from build123d import *

# Parameters (mm, degrees)
F1_DEPTH = 19.05
F2_R     = 50.8
F3_R     = 25.4
F4_R     = 12.7


with BuildPart() as f1:
    # F0 (on Top) → F1 (new body)
    with BuildSketch(Plane.XY):
        Polygon((203.2, 0), (0, 0), (-101.6, 0), (-101.6, -355.6), (-50.8, -355.6), (0, -50.8), (203.2, -50.8), (254, -355.6), (304.8, -355.6), (304.8, 0), align=None)
    extrude(amount=F1_DEPTH)

    # F2
    f2_edges = [f1.edges().sort_by_distance(p)[0] for p in [
        (-101.6, 0, 9.525),
        (304.8, 0, 9.525),
    ]]
    fillet(f2_edges, radius=F2_R)

    # F3
    f3_edges = [f1.edges().sort_by_distance(p)[0] for p in [
        (-101.6, -355.6, 9.525),
        (-50.8, -355.6, 9.525),
        (304.8, -355.6, 9.525),
        (254, -355.6, 9.525),
    ]]
    fillet(f3_edges, radius=F3_R)

    # F4
    f4_edges = [f1.edges().sort_by_distance(p)[0] for p in [
        (203.2, -50.8, 9.525),
        (0, -50.8, 9.525),
    ]]
    fillet(f4_edges, radius=F4_R)


solid = f1.part
Verification items for the finished model (mm, model axes). A direction names the side the tool comes from. Coordinates: 2 decimals unless noted, no trailing zeros. Order: outer loops, then holes, each group sorted by start corner. A loop starts at its lowest first (then second) coordinate and runs counter-clockwise, first axis right, second up. Notation, with made-up numbers: M 13,78 L 69,78 A19 ccw 69,90 Z; hole C 39.25,71.5 d2. An arc over 180 degrees is marked long. Write each question's results on one line, items separated by ' | '.
1) Scan lines: line 1 along X through (y, z) = (-206.5, 3.5); line 2 along X through (y, z) = (-109, 9); line 3 along Y through (x, z) = (123, 14.75). Record each from-to range of solid material in increasing order. Write a range as [from, to].
Solved:
line 1: x = [-101.6, -25.95], [229.15, 304.8] | line 2: x = [-101.6, -9.7], [212.9, 304.8] | line 3: y = [-50.8, 0]
2) Section check C-C on x = -37.5. Record the cut outline in (y, z).
Solved:
outline: M -275.8,0 L 0,0 L 0,19.05 L -275.8,19.05 Z
3) Gauge pin test, flat end, axial feed: pin 1 Ø5.5 at (x, z) = (62, 12) entering from -Y. Record the tip position at first contact, or that the pin passes through.
Solved:
pin 1: stops at y = -50.8
4) Section check D-D on y = -173. Record the cut outline in (x, z).
Solved:
outline: M -101.6,0 L -20.37,0 L -20.37,19.05 L -101.6,19.05 Z; M 223.57,0 L 304.8,0 L 304.8,19.05 L 223.57,19.05 Z
5) Section check B-B on z = 13.25. Record the cut outline in (x, y).
Solved:
outline: M -101.6,-330.2 A25.4 ccw -76.2,-355.6 L -72.32,-355.6 A25.4 ccw -47.26,-334.38 L -1.77,-61.41 A12.7 cw 10.76,-50.8 L 192.44,-50.8 A12.7 cw 204.97,-61.41 L 250.46,-334.38 A25.4 ccw 275.52,-355.6 L 279.4,-355.6 A25.4 ccw 304.8,-330.2 L 304.8,-50.8 A50.8 ccw 254,0 L -50.8,0 A50.8 ccw -101.6,-50.8 Z
6) Section check A-A on y = -269.5. Record the cut outline in (x, z).
Solved:
outline: M -101.6,0 L -36.45,0 L -36.45,19.05 L -101.6,19.05 Z; M 239.65,0 L 304.8,0 L 304.8,19.05 L 239.65,19.05 Z
7) Release check for a two-part mould opening along X. For faces 1 (the face through (-94.36, -347.96, 9.66)), 2 (the face through (2.455, -53.891, 9.658)), 3 (the face through (99, -17, 19.05)), 4 (the face through (304.8, -192, 9)) record: pulls with the +X half, pulls with the -X half, needs draft (parallel to the pull), parting line crosses it, or undercut.
Solved:
face 1: pulls with the -X half | face 2: undercut | face 3: needs draft | face 4: pulls with the +X half
8) Access from +Z, -Z, +X, -X, +Y, -Y to the whole of each face (thin tool, end or side, straight path). Record for faces 5 (the face through (-56.09, -349.74, 9.66)), 6 (the face through (99, -17, 0)).
Solved:
face 5: +Z, -Z, -Y | face 6: -Z, +X, -X, +Y, -Y
